Can you work these out from the drawing? Everything is in mm from the part's minimum corner. A direction names the side the tool comes from. Give positions to 0.01 mm unless a question says otherwise; leave off trailing zeros. Write each loop counter-clockwise with the first axis right and the second up, starting at its lowest first coordinate (ties: lowest second). Pieces come first, ordered by that corner, then holes. Notation, with made-up numbers: (0.25, 13.5) - (46.25, 13.5) arc R20 ccw to (46.25, 39.5) - close; hole circle Ø5 at (15.25, 66.25). An arc over 180 degrees is marked (long way). Return JSON: item names as keys, results as strings. Group by question number.
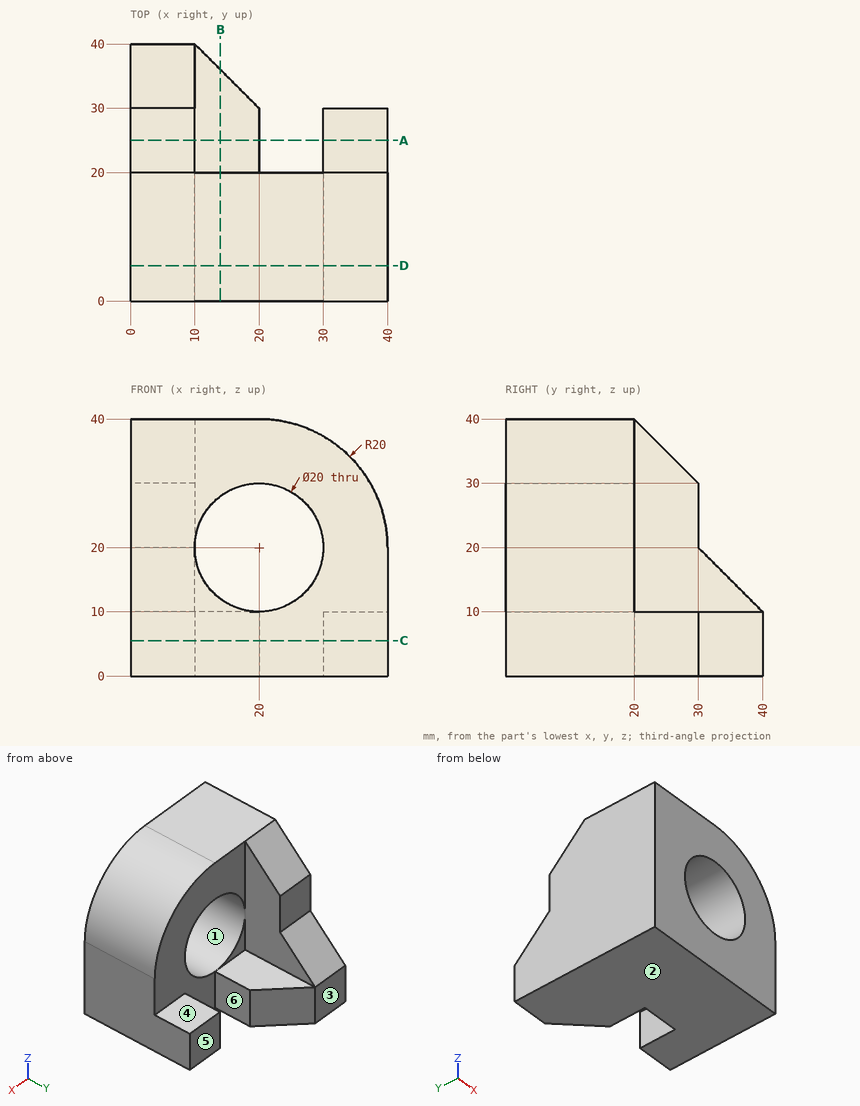
1) Imagine slicing it at C-C, the plane z = 5.5. Write out the boundary of the cut face in (x, y).
2) Imagine slicing it at B-B, the plane x = 14. Write out the boundary of the cut face in (y, z), and give its area (3 significant figures).
3) I need wall thicknesses on line 1 along Y through (x, z) = (5.5, 25); line 2 along X through (y, z) = (14.5, 28.5); line 3 along Z through (x, y) = (16.5, 10). Which ranges of each line are inside material? Lowest first, please.
4) We'd pull the mould along Z, two halves only. Please class the marked faces 1, 2 and 3: pulls with the +Z half, pulls with the -Z half, needs draft (parallel to the pull), parting line crosses it, or undercut.
5) On a 3-axis mill with a long thin cutter (end or side, diameter ignored), from which of +Z, -Z, +X, -X, +Y, -Y can I reach the whole of each face in a straight line? I mean the marked faces 4, 5 and 6. Say none if no direction works.
6) Imagine slicing it at A-A, the plane y = 25. Write out the boundary of the cut face in (x, z).
7) Will these pins go through, and if not, where does the flat tip stop? pin 1 Ø5 at (x, y) = (32.5, 25.5) entering from +Z; pin 2 Ø8 at (x, y) = (26, 8) entering from +Z; pin 3 Ø5 at (x, z) = (36, 4.5) entering from +Y.
8) Imagine slicing it at D-D, the plane y = 5.5. Write out the boundary of the cut face in (x, z), and give its area (3 significant figures).
Resolved:
{
 "1": {"outline": "(0, 0) - (40, 0) - (40, 30) - (30, 30) - (30, 20) - (20, 20) - (20, 30) - (10, 40) - (0, 40) - close"},
 "2": {"outline": "(0, 0) - (36, 0) - (36, 10) - (20, 10) - (20, 12) - (0, 12) - close; (0, 28) - (20, 28) - (20, 40) - (0, 40) - close", "area": "640 mm^2"},
 "3": {"line 1": "0 to 30", "line 2": "0 to 14.73, 25.27 to 38.1", "line 3": "0 to 10.63, 29.37 to 40"},
 "4": {"face 1": "undercut", "face 2": "pulls with the -Z half", "face 3": "needs draft"},
 "5": {"face 4": "+Z, +X, +Y", "face 5": "+Z, -Z, +X, +Y", "face 6": "+Z, -Z, +Y"},
 "6": {"outline": "(0, 0) - (20, 0) - (20, 10) - (10, 10) - (10, 35) - (0, 35) - close; (30, 0) - (40, 0) - (40, 10) - (30, 10) - close"},
 "7": {"pin 1": "z = 10", "pin 2": "z = 39.9", "pin 3": "y = 30"},
 "8": {"outline": "(0, 0) - (40, 0) - (40, 20) arc R20 ccw to (20, 40) - (0, 40) - close; hole circle Ø20 at (20, 20)", "area": "1,200 mm^2"}
}
